Here's how the part is built. I have some questions about the finished solid (model axes, mm). A direction names the side the tool comes from. Give positions to 0.01 mm unless a question says otherwise; leave off trailing zeros. Loops run counter-clockwise (first coordinate to the right, second up) from the corner with the lowest first, then second, coordinate; pieces in that order, holes last.
Q1. If we section it at C-C (z = 37.5): Please give me the cut outline in (x, y).
Q2. Will these pins go through, and if not, where does the flat tip stop? P1, Ø3, axis at x = -4.5, z = 9.5, coming from the -Y side; P2, Ø12, axis at x = 19, y = -18, coming from the +Z side; P3, Ø2, axis at y = -2, z = 25, coming from the -X side.
Q3. If we section it at D-D (x = 11.5): Please give me the cut outline in (y, z), plus the area to 3 significant figures.
Q4. For faces 1 (the face through (-1, 1, 0)), 2 (the face through (3.2, 1.8, 10)), which set-ups out of +Z, -Z, +X, -X, +Y, -Y let a thin tool reach every point of the face, with its end or its side?
Q5. I need wall thicknesses on line 1 (Z direction, x = -5, y = 30.5); line 2 (Y direction, x = -0.5, z = 31); line 3 (X direction, y = 1, z = 33). Which ranges of each line are inside material? Lowest first, please.
Q6. If we section it at A-A (x = 0): Please give me the cut outline in (y, z), plus the area to 3 significant figures.
from build123d import *

# Parameters (mm, degrees)
CYLINDER002_R     = 3.5
CYLINDER002_DEPTH = 30
CYLINDER001_R     = 7.5
CYLINDER001_DEPTH = 5
CYLINDER_R        = 40
CYLINDER_DEPTH    = 5


with BuildPart() as cilindro:
    # Cylinder002 → Cylinder002 (new body)
    with BuildSketch(Plane.XY.offset(10)):
        Circle(CYLINDER002_R)
    extrude(amount=CYLINDER002_DEPTH)


with BuildPart() as obj1:
    # Cylinder001 → Cylinder001 (new body)
    with BuildSketch(Plane.XY.offset(5)):
        Circle(CYLINDER001_R)
    extrude(amount=CYLINDER001_DEPTH)


with BuildPart() as fusion001:
    # Cylinder → Cylinder (new body)
    with BuildSketch(Plane.XY):
        Circle(CYLINDER_R)
    extrude(amount=CYLINDER_DEPTH)

    # Fusion: union obj1
    add(obj1.part)

    # Fusion001: union Cilindro
    add(cilindro.part)


solid = fusion001.part
Check sheet entries:
1. outline: circle Ø7 at (0, 0)
2. P1: stops at y = -6.87
2. P2: stops at z = 5
2. P3: stops at x = -3.35
3. outline: (-38.31, 0) - (38.31, 0) - (38.31, 5) - (-38.31, 5) - close
3. area: 383 mm2
4. face 1: -Z, +X, -X, +Y, -Y
4. face 2: +Z
5. line 1: z = 0 to 5
5. line 2: y = -3.46 to 3.46
5. line 3: x = -3.35 to 3.35
6. outline: (-40, 0) - (40, 0) - (40, 5) - (7.5, 5) - (7.5, 10) - (3.5, 10) - (3.5, 40) - (-3.5, 40) - (-3.5, 10) - (-7.5, 10) - (-7.5, 5) - (-40, 5) - close
6. area: 685 mm2
